```python
from build123d import *

# Parameters (mm, degrees)
F0_W     = 812.8
F0_H     = 584.2
F1_DEPTH = 2235.2
F2_W     = 152.4
F2_H     = 76.2
F2_W_2   = 508
F2_W_3   = 50.8
F3_DEPTH = 2235.201
F4_W     = 711.2
F4_H     = 406.4
F5_DEPTH = 2235.201
F6_W     = 2133.6
F6_H     = 482.6
F7_DEPTH = 812.801
F8_W     = 279.4
F8_H     = 2133.6
F9_DEPTH = 25.4


with BuildPart() as f1:
    # F0 (on Front) → F1 (new body)
    with BuildSketch(Plane.XZ):
        with Locations((-406.4, 292.1)):
            Rectangle(F0_W, F0_H)
    extrude(amount=F1_DEPTH)

    # F2 (on face) → F3 (cut, through all)
    with BuildSketch(Plane.XZ.offset(2235.2)):
        with Locations((-736.6, 546.1)):
            Rectangle(F2_W, F2_H)
        with Locations((-355.6, 546.1)):
            Rectangle(F2_W_2, F2_H)
        with Locations((-25.4, 546.1)):
            Rectangle(F2_W_3, F2_H)
    extrude(amount=-F3_DEPTH, mode=Mode.SUBTRACT)

    # F4 (on face) → F5 (cut, through all)
    with BuildSketch(Plane.XZ.offset(2235.2)):
        with Locations((-406.4, 254)):
            Rectangle(F4_W, F4_H)
    extrude(amount=-F5_DEPTH, mode=Mode.SUBTRACT)

    # F6 (on face) → F7 (cut, through all)
    with BuildSketch(Plane.YZ):
        with Locations((-1117.6, 266.7)):
            Rectangle(F6_W, F6_H)
    extrude(amount=-F7_DEPTH, mode=Mode.SUBTRACT)

    # F8 (on face) → F9 (cut)
    with BuildSketch(Plane.XY.offset(25.4)):
        with Locations((-139.7, -1117.6)):
            Rectangle(F8_W, F8_H)
    extrude(amount=-F9_DEPTH, mode=Mode.SUBTRACT)


solid = f1.part
```
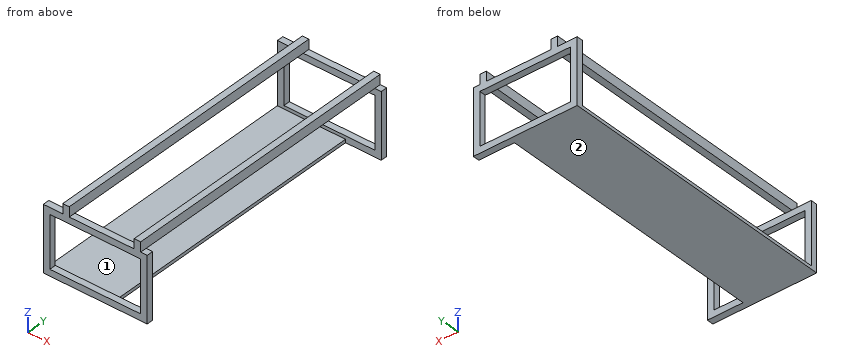
Verification items for the finished model (mm, model axes). Face numbers are marked on the shaded views. Round coordinates to 2 decimals unless told otherwise and drop trailing zeros. Write each loop counter-clockwise with the first axis right and the second up, starting at its lowest first coordinate (ties: lowest second). Pieces come first, ordered by that corner, then holes.
1. Section check B-B on z = 434. Enter the section's corners in (x, y), plus the area to 3 significant figures.
2. Gauge pin test, flat ends, axial feed: P1, Ø6, axis at x = -279.5, y = -1670, coming from the +Z side; P2, Ø23, axis at y = -785.5, z = 542, coming from the +X side; P3, Ø23, axis at y = -767.5, z = 550, coming from the -X side. Record the tip position at first contact, or that the pin passes through.
3. Draft check along Y on the marked faces 1 and 2. Enter one of: +Y half, -Y half, draft (parallel to the pull), parting line (faces both ways), or undercut.
4. Scan lines: L1, parallel to Y at x = -42.5, z = 364; L2, parallel to X at y = -1732.5, z = 534; L3, parallel to Z at x = -370, y = -850.5. Record each from-to range of solid material in increasing order.
5. Section check A-A on y = -806.5. Enter the section's corners in (x, z), plus the area to 3 significant figures.
6. Section check D-D on x = -570.5. Enter the section's corners in (y, z).
7. Section check C-C on x = -175. Enter the section's corners in (y, z), plus the area to 3 significant figures.
Answer:
1. outline: (-812.8, -2235.2) - (-762, -2235.2) - (-762, -2184.4) - (-812.8, -2184.4) - close; (-812.8, -50.8) - (-762, -50.8) - (-762, 0) - (-812.8, 0) - close; (-50.8, -2235.2) - (0, -2235.2) - (0, -2184.4) - (-50.8, -2184.4) - close; (-50.8, -50.8) - (0, -50.8) - (0, 0) - (-50.8, 0) - close
1. area: 10,300 mm2
2. P1: stops at z = 25.4
2. P2: stops at x = -50.8
2. P3: stops at x = -660.4
3. face 1: undercut
3. face 2: draft
4. L1: y = -2235.2 to -2184.4, -50.8 to 0
4. L2: x = -660.4 to -609.6, -101.6 to -50.8
4. L3: z = 0 to 25.4
5. outline: (-812.8, 0) - (-279.4, 0) - (-279.4, 25.4) - (-812.8, 25.4) - close; (-660.4, 508) - (-609.6, 508) - (-609.6, 584.2) - (-660.4, 584.2) - close; (-101.6, 508) - (-50.8, 508) - (-50.8, 584.2) - (-101.6, 584.2) - close
5. area: 21,300 mm2
6. outline: (-2235.2, 0) - (0, 0) - (0, 50.8) - (-50.8, 50.8) - (-50.8, 25.4) - (-2184.4, 25.4) - (-2184.4, 50.8) - (-2235.2, 50.8) - close; (-2235.2, 457.2) - (-2184.4, 457.2) - (-2184.4, 508) - (-2235.2, 508) - close; (-50.8, 457.2) - (0, 457.2) - (0, 508) - (-50.8, 508) - close
7. outline: (-2235.2, 0) - (-2184.4, 0) - (-2184.4, 50.8) - (-2235.2, 50.8) - close; (-2235.2, 457.2) - (-2184.4, 457.2) - (-2184.4, 508) - (-2235.2, 508) - close; (-50.8, 0) - (0, 0) - (0, 50.8) - (-50.8, 50.8) - close; (-50.8, 457.2) - (0, 457.2) - (0, 508) - (-50.8, 508) - close
7. area: 10,300 mm2
